```python
from build123d import *

# Parameters (mm, degrees)
SKETCH1_R                = 3.3
BOSS_EXTRUDE1_DEPTH      = 1.83
BOSS_EXTRUDE2_DEPTH      = 9.51
BOSS_EXTRUDE2_DEPTH_BACK = 9.51


with BuildPart() as part:
    # Sketch1 → Boss-Extrude1 (new body)
    with BuildSketch(Plane(origin=(0, 0, 0), x_dir=(1, 0, 0), z_dir=(0, 1, 0))):
        with BuildLine():
            Line((-32.29, 8.13), (32.29, 8.13))
            ThreePointArc((32.29, 8.13), (33.704213562, 7.544213562), (34.29, 6.13))
            Line((34.29, 6.13), (34.29, -6.13))
            ThreePointArc((34.29, -6.13), (33.704213562, -7.544213562), (32.29, -8.13))
            Line((32.29, -8.13), (-32.29, -8.13))
            ThreePointArc((-32.29, -8.13), (-33.704213562, -7.544213562), (-34.29, -6.13))
            Line((-34.29, -6.13), (-34.29, 6.13))
            ThreePointArc((-34.29, 6.13), (-33.704213562, 7.544213562), (-32.29, 8.13))
        make_face()
        with Locations((25.4, 0)):
            Circle(SKETCH1_R, mode=Mode.SUBTRACT)
        with Locations((-25.4, 0)):
            Circle(SKETCH1_R, mode=Mode.SUBTRACT)
    extrude(amount=BOSS_EXTRUDE1_DEPTH)

    # Sketch2 → Boss-Extrude2 (add, two sides)
    with BuildSketch(Plane.XY) as boss_extrude2_sk:
        Polygon((-14.6, 3.275), (-11.6, 6.275), (11.6, 6.275), (14.6, 3.275), (14.6, -1.445), (11.6, -4.445), (-11.6, -4.445), (-14.6, -1.445), align=None)
    extrude(amount=BOSS_EXTRUDE2_DEPTH)
    extrude(boss_extrude2_sk.sketch, amount=-BOSS_EXTRUDE2_DEPTH_BACK)


solid = part.part
```
Source: CAD feature listing. Evaluate the final solid. Frame: model axes, mm. A direction names the side the tool comes from. Give positions to 0.01 mm unless a question says otherwise; leave off trailing zeros. Loops run counter-clockwise (first coordinate to the right, second up) from the corner with the lowest first, then second, coordinate; pieces in that order, holes last. Notation, with made-up numbers: (-1, 60.5) -> (44, 60.5) arc R24 ccw to (44, 81.5) -> close; hole circle Ø10 at (-35, 57). An arc over 180 degrees is marked (long way). Use a Markdown table: item, result. Add a question column.
(1) Ray query, line 1 (X direction, y = 0.9, z = 0); line 2 (Z direction, x = 25.4, y = 1.35); line 3 (Y direction, x = 30.5, z = -7.25). Return the intervals inside material, ascending.
(2) Section query D-D (x = 16). Output: boundary loops of the cut face in (y, z).
(3) Section query B-B (x = -25.4). Output: boundary loops of the cut face in (y, z).
(4) First-contact query: pin 1 Ø1.5 at (y, z) = (4, -2) entering from +X; pin 2 Ø0.9 at (x, y) = (-24, 0.5) entering from +Z; pin 3 Ø0.9 at (x, y) = (21, 1) entering from -Z; pin 4 Ø4 at (x, z) = (-25.4, 0) entering from +Y. Flat tips, straight axial feed; report the tip coordinate or a pass-through.
(5) Access query for faces 4 (the face through (22, 0, -2)), 5 (the face through (22, 1.83, -2)), 6 (the face through (-23, 1, 8.13)). Directions: +Z, -Z, +X, -X, +Y, -Y. A direction counts if a zero-diameter tool reaches every point of the face in a straight line with its end or side. Return the directions, or none.
(6) Pull-direction query (X, two-part tool) for faces 1 (the face through (-22, 0, -2)), 2 (the face through (-22.35, 0.9, 1.26)), 3 (the face through (13.079, 4.796, 0.133)); classes: +X half, -X half, draft (parallel to the pull), parting line (faces both ways), or undercut.
(7) Section query A-A (z = 0). Output: boundary loops of the cut face in (x, y) (3 decimals), then the cut area to 3 significant figures.
(8) Section query C-C (z = 4.5). Output: boundary loops of the cut face in (x, y) (3 decimals), then the cut area to 3 significant figures.
Checked values:
| question | item | result |
|---|---|---|
| 1 | line 1 | -34.29 to -28.7, -22.1 to 22.1, 28.7 to 34.29 |
| 1 | line 2 | -8.13 to -3.3, 3.3 to 8.13 |
| 1 | line 3 | 0 to 1.83 |
| 2 | outline | (0, -8.13) -> (1.83, -8.13) -> (1.83, 8.13) -> (0, 8.13) -> close |
| 3 | outline | (0, -8.13) -> (1.83, -8.13) -> (1.83, -3.3) -> (0, -3.3) -> close; (0, 3.3) -> (1.83, 3.3) -> (1.83, 8.13) -> (0, 8.13) -> close |
| 4 | pin 1 | x = 14.6 |
| 4 | pin 2 | z = 8.13 |
| 4 | pin 3 | z = -8.13 |
| 4 | pin 4 | through |
| 5 | face 4 | +Z, -Z, +X, -Y |
| 5 | face 5 | +Z, -Z, +X, +Y |
| 5 | face 6 | +Z, -X, +Y, -Y |
| 6 | face 1 | draft |
| 6 | face 2 | undercut |
| 6 | face 3 | +X half |
| 7 | outline | (-34.29, 0) -> (-28.7, 0) -> (-28.7, 1.83) -> (-34.29, 1.83) -> close; (-22.1, 0) -> (-14.6, 0) -> (-14.6, -1.445) -> (-11.6, -4.445) -> (11.6, -4.445) -> (14.6, -1.445) -> (14.6, 0) -> (22.1, 0) -> (22.1, 1.83) -> (14.6, 1.83) -> (14.6, 3.275) -> (11.6, 6.275) -> (-11.6, 6.275) -> (-14.6, 3.275) -> (-14.6, 1.83) -> (-22.1, 1.83) -> close; (28.7, 0) -> (34.29, 0) -> (34.29, 1.83) -> (28.7, 1.83) -> close |
| 7 | area | 343 mm^2 |
| 8 | outline | (-34.29, 0) -> (-14.6, 0) -> (-14.6, -1.445) -> (-11.6, -4.445) -> (11.6, -4.445) -> (14.6, -1.445) -> (14.6, 0) -> (34.29, 0) -> (34.29, 1.83) -> (14.6, 1.83) -> (14.6, 3.275) -> (11.6, 6.275) -> (-11.6, 6.275) -> (-14.6, 3.275) -> (-14.6, 1.83) -> (-34.29, 1.83) -> close |
| 8 | area | 367 mm^2 |
